```python
from build123d import *

# Parameters (mm, degrees)
F0_R     = 20
F1_DEPTH = 125
F2_R     = 7.5
F3_DEPTH = 25
F4_R     = 20
F5_DEPTH = 10
F5_TAPER = -45
F6_R     = 40
F6_R_2   = 30
F7_DEPTH = 10
F7_TAPER = 45
F8_SIZE2 = 3
F8_SIZE  = 3


with BuildPart() as f1:
    # F0 (on Top) → F1 (new body)
    with BuildSketch(Plane.XY):
        Circle(F0_R)
    extrude(amount=F1_DEPTH)

    # F2 (on face) → F3 (join)
    with BuildSketch(Plane.XY.offset(125)):
        Circle(F2_R)
    extrude(amount=F3_DEPTH)

    # F4 (on face) → F5 (join)
    with BuildSketch(Plane(origin=(0, 0, 0), x_dir=(1, 0, 0), z_dir=(0, 0, -1))):
        Circle(F4_R)
    extrude(amount=F5_DEPTH, taper=F5_TAPER)

    # F6 (on face) → F7 (join)
    with BuildSketch(Plane(origin=(0, 0, -10), x_dir=(1, 0, 0), z_dir=(0, 0, -1))):
        Circle(F6_R)
        Circle(F6_R_2, mode=Mode.SUBTRACT)
        Circle(F6_R_2)
    extrude(amount=F7_DEPTH, taper=F7_TAPER)

    # F8
    f8_edges = [f1.edges().sort_by_distance(p)[0] for p in [
        (-20, 0, 125),
    ]]
    chamfer(f8_edges, length=F8_SIZE, length2=F8_SIZE2)


solid = f1.part
```
The listing builds one solid part. Answer for the finished solid, in the listing's coordinates (mm). A direction names the side the tool comes from. Coordinates: 2 decimals unless noted, no trailing zeros. Write each loop counter-clockwise with the first axis right and the second up, starting at its lowest first coordinate (ties: lowest second). Pieces come first, ordered by that corner, then holes. Notation, with made-up numbers: (-1, 18.25) - (55, 18.25) arc R18 cw to (55, 40.25) - close; hole circle Ø4 at (-37.75, -22.75). An arc over 180 degrees is marked (long way). Return JSON: item names as keys, results as strings. Group by question number.
Q1. The part is cut by section C-C on z = 72.5. Write down the section's boundary in (x, y).
Q2. The part is cut by section A-A on x = 0. Write down the section's boundary in (y, z).
Q3. The part is cut by section B-B on z = 129. Write down the section's boundary in (x, y).
Q4. Find the intervals of material crossed by line 1 along Z through (x, y) = (4.5, 7); line 2 along Y through (x, z) = (-10.5, 56); line 3 along Z through (x, y) = (17.5, -28), in increasing order. Write a range as [from, to].
Q5. Which of the six approach directions +Z, -Z, +X, -X, +Y, -Y give full straight-line access (tool end or side, diameter ignored) to faces 1 (the flat face through (0, 0, -20)), 2 (the flat face through (7, -4, 125))?
Q6. Flat-ended cylindrical pins translate along their axes: pin 1 Ø1 at (x, y) = (-19, -7) entering from +Z; pin 2 Ø6 at (x, y) = (16, -9) entering from +Z; pin 3 Ø12 at (y, z) = (-30.5, 92.5) entering from +X; pin 4 Ø12 at (y, z) = (5.5, 121.5) entering from -X. Find the tip coordinate at first contact, or state that the pin passes through.
Evaluation:
{
 "1": {"outline": "circle Ø40 at (0, 0)"},
 "2": {"outline": "(-40, -10) - (-30, -20) - (30, -20) - (40, -10) - (30, -10) - (20, 0) - (20, 122) - (17, 125) - (7.5, 125) - (7.5, 150) - (-7.5, 150) - (-7.5, 125) - (-17, 125) - (-20, 122) - (-20, 0) - (-30, -10) - close"},
 "3": {"outline": "circle Ø15 at (0, 0)"},
 "4": {"line 1": "z = [-20, 125]", "line 2": "y = [-17.02, 17.02]", "line 3": "z = [-16.98, -10]"},
 "5": {"face 1": "-Z, +X, -X, +Y, -Y", "face 2": "+Z"},
 "6": {"pin 1": "stops at z = 122.25", "pin 2": "stops at z = 125", "pin 3": "passes through", "pin 4": "stops at x = -20"}
}
